Could you check a few things on this model? Use its own coordinates, in mm. Coordinates: 2 decimals unless noted, no trailing zeros. Write each loop counter-clockwise with the first axis right and the second up, starting at its lowest first coordinate (ties: lowest second). Pieces come first, ordered by that corner, then holes. Notation, with made-up numbers: (-6.75, 59.5) - (46.25, 59.5) arc R24 ccw to (46.25, 91.5) - close; hole circle Ø5 at (-28, 82.25). An arc over 180 degrees is marked (long way). Answer as a JSON object with one key per item and string values. Group by question number.
1) Will these pins go through, and if not, where does the flat tip stop? pin 1 Ø1.5 at (y, z) = (21, 1) entering from -X; pin 2 Ø8 at (x, y) = (16.5, 12.5) entering from +Z; pin 3 Ø1.5 at (x, z) = (23, 2) entering from -Y; pin 4 Ø0.9 at (y, z) = (21, 2) entering from +X.
2) If we section it at B-B (y = -10): Write out the boundary of the cut face in (x, z).
3) If we section it at C-C (x = 10.5): Write out the boundary of the cut face in (y, z).
4) Please list where these lines run through material, in increasing order: line 1 along X through (y, z) = (-14, 2.5); line 2 along X through (y, z) = (4.5, 2.65); line 3 along Y through (x, z) = (15, 2.7).
5) If we section it at D-D (z = 2.55): State how many separate pieces and enclosed holes the cut face has, plus the area to 3 significant figures.
6) If we section it at A-A (y = 10): Write out the boundary of the cut face in (x, z), plus the area to 3 significant figures.
```python
from build123d import *

# Parameters (mm, degrees)
SKETCH1_R           = 1
SKETCH1_R_2         = 8.4
BOSS_EXTRUDE1_DEPTH = 3
SKETCH2_W           = 7
SKETCH2_H           = 4
BOSS_EXTRUDE2_DEPTH = 3
SKETCH5_W           = 3
SKETCH5_H           = 36.4
BOSS_EXTRUDE3_DEPTH = 3
FILLET2_R           = 2.5
FILLET3_R           = 1


with BuildPart() as part:
    # Sketch1 → Boss-Extrude1 (new body)
    with BuildSketch(Plane.XY):
        with BuildLine():
            Line((-20.667019059, -16.4), (-20.667019059, 20))
            Line((-20.667019059, 20), (-15.667019059, 20))
            Line((-15.667019059, 20), (-15.667019059, 23))
            Line((-15.667019059, 23), (-10.667019059, 23))
            Line((-10.667019059, 23), (-10.667019059, 20))
            Line((-10.667019059, 20), (-3.167019059, 20))
            Line((-3.167019059, 20), (-3.167019059, 15.5))
            Line((-3.167019059, 15.5), (6.832980941, 15.5))
            Line((6.832980941, 15.5), (6.832980941, 20))
            Line((6.832980941, 20), (14.332980941, 20))
            Line((14.332980941, 20), (14.332980941, 23))
            Line((14.332980941, 23), (19.332980941, 23))
            Line((19.332980941, 23), (19.332980941, 20))
            Line((19.332980941, 20), (24.332980941, 20))
            Line((24.332980941, 20), (24.332980941, -16.4))
            Line((24.332980941, -16.4), (21.832980941, -16.4))
            Line((21.832980941, -16.4), (21.832980941, -19.4))
            Line((21.832980941, -19.4), (16.832980941, -19.4))
            Line((16.832980941, -19.4), (16.832980941, -16.4))
            Line((16.832980941, -16.4), (14.332980941, -16.4))
            Line((14.332980941, -16.4), (14.332980941, -1))
            ThreePointArc((14.332980941, -1), (14.040087722, -0.292893219), (13.332980941, 0))
            Line((13.332980941, 0), (7.332980941, 0))
            Line((7.332980941, 0), (7.332980941, 2))
            Line((7.332980941, 2), (-3.667019059, 2))
            Line((-3.667019059, 2), (-3.667019059, 0))
            Line((-3.667019059, 0), (-9.667019059, 0))
            ThreePointArc((-9.667019059, 0), (-10.37412584, -0.292893219), (-10.667019059, -1))
            Line((-10.667019059, -1), (-10.667019059, -16.4))
            Line((-10.667019059, -16.4), (-13.167019059, -16.4))
            Line((-13.167019059, -16.4), (-13.167019059, -19.4))
            Line((-13.167019059, -19.4), (-18.167019059, -19.4))
            Line((-18.167019059, -19.4), (-18.167019059, -16.4))
            Line((-18.167019059, -16.4), (-20.667019059, -16.4))
        make_face()
        with Locations((22.332980941, 18)):
            Circle(SKETCH1_R, mode=Mode.SUBTRACT)
        with Locations((-18.667019059, 2)):
            Circle(SKETCH1_R, mode=Mode.SUBTRACT)
        with Locations((-10.867019059, 10)):
            Circle(SKETCH1_R_2, mode=Mode.SUBTRACT)
        with Locations((14.532980941, 10)):
            Circle(SKETCH1_R_2, mode=Mode.SUBTRACT)
    extrude(amount=BOSS_EXTRUDE1_DEPTH)

    # Sketch2 → Boss-Extrude2 (add)
    with BuildSketch(Plane.XY.offset(3)):
        with Locations((-7.167019059, -1)):
            Rectangle(SKETCH2_W, SKETCH2_H)
        with Locations((10.832980941, -1)):
            Rectangle(SKETCH2_W, SKETCH2_H)
    extrude(amount=-BOSS_EXTRUDE2_DEPTH)

    # Sketch5 → Boss-Extrude3 (add)
    with BuildSketch(Plane(origin=(24.332980941, 0, 0), x_dir=(0, 0, -1), z_dir=(1, 0, 0))):
        with Locations((-1.5, 1.8)):
            Rectangle(SKETCH5_W, SKETCH5_H)
    boss_extrude3 = extrude(amount=BOSS_EXTRUDE3_DEPTH)

    # Mirror1: Boss-Extrude3 across plane
    add(boss_extrude3.mirror(Plane(origin=(1.832980941, 0, 0), x_dir=(0, 0, 1), z_dir=(1, 0, 0))))

    # Fillet2
    fillet2_edges = [part.edges().sort_by_distance(p)[0] for p in [
        (-10.667019059, -3, 1.5),
        (-3.667019059, -3, 1.5),
        (7.332980941, -3, 1.5),
        (14.332980941, -3, 1.5),
        (27.332980941, -16.4, 1.5),
        (27.332980941, 20, 1.5),
        (-23.667019059, 20, 1.5),
        (-23.667019059, -16.4, 1.5),
        (-3.167019059, 15.5, 1.5),
        (6.832980941, 15.5, 1.5),
    ]]
    fillet(fillet2_edges, radius=FILLET2_R)

    # Fillet3
    fillet3_edges = [part.edges().sort_by_distance(p)[0] for p in [
        (7.332980941, 2, 1.5),
        (-3.667019059, 2, 1.5),
    ]]
    fillet(fillet3_edges, radius=FILLET3_R)


solid = part.part
```
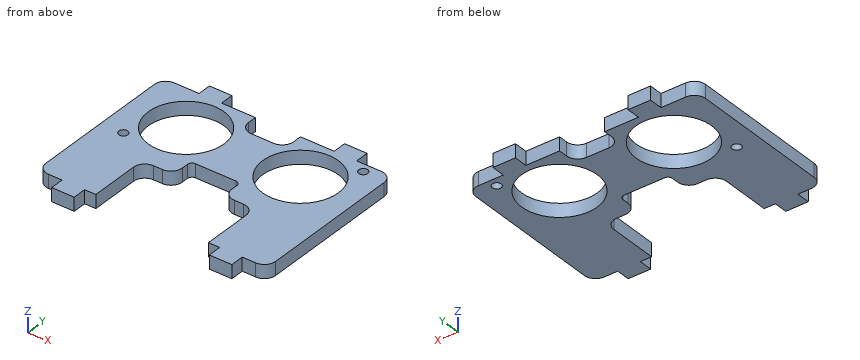
Here are the results:
{
 "1": {"pin 1": "stops at x = -15.67", "pin 2": "passes through", "pin 3": "stops at y = -16.4", "pin 4": "stops at x = 19.33"},
 "2": {"outline": "(-23.67, 0) - (-10.67, 0) - (-10.67, 3) - (-23.67, 3) - close; (14.33, 0) - (27.33, 0) - (27.33, 3) - (14.33, 3) - close"},
 "3": {"outline": "(-3, 0) - (2.63, 0) - (2.63, 3) - (-3, 3) - close; (17.37, 0) - (20, 0) - (20, 3) - (17.37, 3) - close"},
 "4": {"line 1": "x = -23.67 to -10.67, 14.33 to 27.33", "line 2": "x = -23.67 to -17.22, -4.52 to 8.18, 20.88 to 27.33", "line 3": "y = -16.4 to 1.61, 18.39 to 23"},
 "5": {"separate pieces": "1", "enclosed holes": "4", "area": "1,030 mm²"},
 "6": {"outline": "(-23.67, 0) - (-19.27, 0) - (-19.27, 3) - (-23.67, 3) - close; (-2.47, 0) - (6.13, 0) - (6.13, 3) - (-2.47, 3) - close; (22.93, 0) - (27.33, 0) - (27.33, 3) - (22.93, 3) - close", "area": "52.2 mm²"}
}
